Can you work these out from the drawing? Everything is in mm from the part's minimum corner. A direction names the side the tool comes from. Give positions to 0.01 mm unless a question says otherwise; leave off trailing zeros. Loops run counter-clockwise (first coordinate to the right, second up) from the corner with the lowest first, then second, coordinate; pieces in that order, holes last. Notation, with made-up numbers: (5.5, 62.5) - (28.5, 62.5) arc R24 ccw to (28.5, 100.5) - close; hole circle Ø5 at (52.5, 39.25). An arc over 180 degrees is marked (long way). Answer in a Markdown table with one row per item.
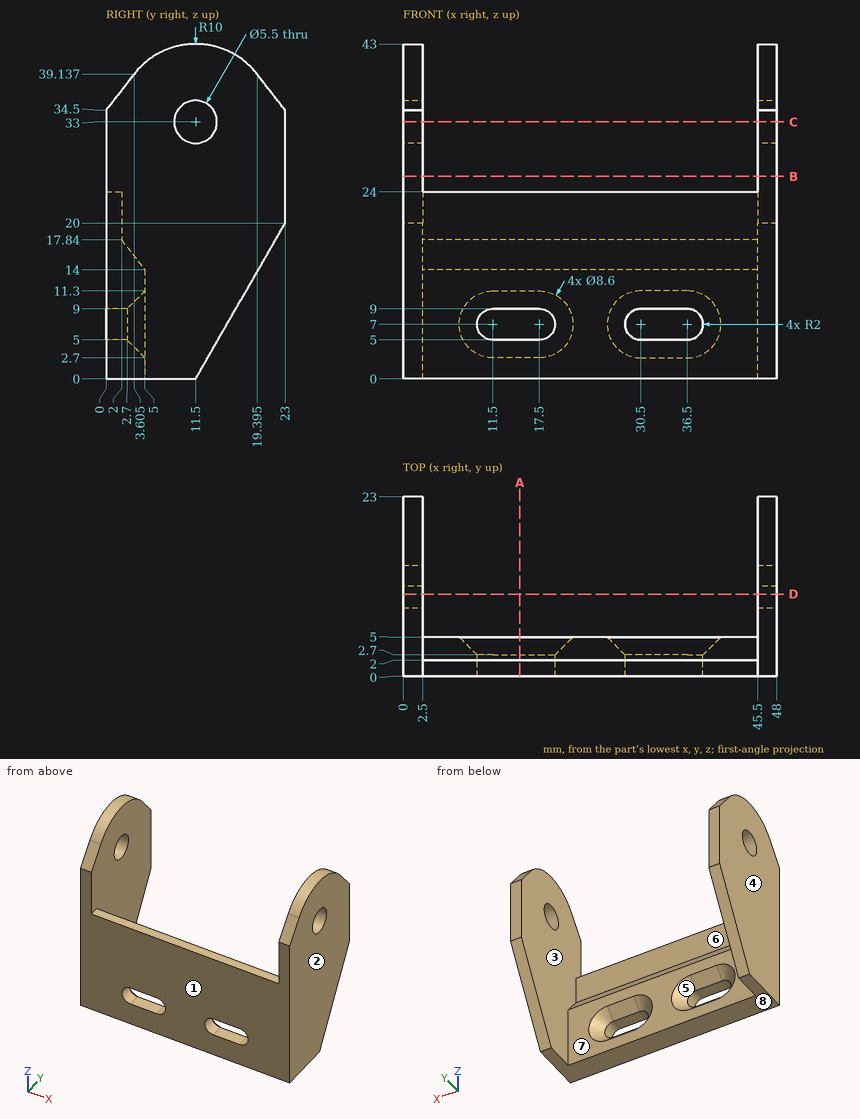
Q1. Imagine slicing it at B-B, the plane z = 26. Write out the boundary of the cut face in (x, y).
Checked values:
| item | result |
|---|---|
| outline | (0, 0) - (2.5, 0) - (2.5, 23) - (0, 23) - close; (45.5, 0) - (48, 0) - (48, 23) - (45.5, 23) - close |
Q2. On a 3-axis mill with a long thin cutter (end or side, diameter ignored), from which of +Z, -Z, +X, -X, +Y, -Y can I reach the whole of each face in a straight line? I mean the marked faces 5, 6, 7 and 8. Say none if no direction works.
Checked values:
| item | result |
|---|---|
| face 5 | +Y |
| face 6 | +Z, +Y |
| face 7 | +Z, -Z, +Y |
| face 8 | -Z, +X, -X, +Y, -Y |
Q3. If we mould it in two halves opening along X, with no side actions, what happens to the marked faces 1, 2, 3 and 4? For each: released by +X, released by -X, zero draft, split by the parting line, or undercut.
Checked values:
| item | result |
|---|---|
| face 1 | zero draft |
| face 2 | released by +X |
| face 3 | undercut |
| face 4 | released by -X |
Q4. Imagine slicing it at C-C, the plane z = 33. Write out the boundary of the cut face in (x, y).
Checked values:
| item | result |
|---|---|
| outline | (0, 0) - (2.5, 0) - (2.5, 8.75) - (0, 8.75) - close; (0, 14.25) - (2.5, 14.25) - (2.5, 23) - (0, 23) - close; (45.5, 0) - (48, 0) - (48, 8.75) - (45.5, 8.75) - close; (45.5, 14.25) - (48, 14.25) - (48, 23) - (45.5, 23) - close |
Q5. For pin 1 (10 mm diameter, centred on x = 8, y = 13, fed in from +Z); pin 2 (6 mm diameter, centred on x = 16, z = 6.5, fed in from -Y); pin 3 (5 mm diameter, centred on x = 19, z = 21, fed in from +Y); pin 4 (11 mm diameter, centred on x = 31, z = 6, fed in from +Y), each with a flat end and sliding along its axis, tell me the tip position at first contact or that it passes through.
Checked values:
| item | result |
|---|---|
| pin 1 | passes through |
| pin 2 | stops at y = 0 |
| pin 3 | stops at y = 2 |
| pin 4 | stops at y = 5 |
Q6. Imagine slicing it at A-A, the plane x = 15. Write out the boundary of the cut face in (y, z).
Checked values:
| item | result |
|---|---|
| outline | (0, 0) - (5, 0) - (5, 2.7) - (2.7, 5) - (0, 5) - close; (0, 9) - (2.7, 9) - (5, 11.3) - (5, 14) - (2, 17.84) - (2, 24) - (0, 24) - close |
Q7. If I drill on line 1 (X direction, y = 1.5, z = 7); line 2 (X direction, y = 9.25, z = 37); line 3 (Y direction, x = 1.1, z = 33), over which ranges is the centre line in solid material (lowest first)? Write a range as [from, to].
Checked values:
| item | result |
|---|---|
| line 1 | x = [0, 9.5], [19.5, 28.5], [38.5, 48] |
| line 2 | x = [0, 2.5], [45.5, 48] |
| line 3 | y = [0, 8.75], [14.25, 23] |
Q8. Imagine slicing it at D-D, the plane y = 10.5. Write out the boundary of the cut face in (x, z).
Checked values:
| item | result |
|---|---|
| outline | (0, 0) - (2.5, 0) - (2.5, 30.44) - (0, 30.44) - close; (0, 35.56) - (2.5, 35.56) - (2.5, 42.95) - (0, 42.95) - close; (45.5, 0) - (48, 0) - (48, 30.44) - (45.5, 30.44) - close; (45.5, 35.56) - (48, 35.56) - (48, 42.95) - (45.5, 42.95) - close |
